from build123d import *

# Parameters (mm, degrees)
F0_R     = 1
F0_R_2   = 1.524
F1_DEPTH = 6.35


with BuildPart() as f1:
    # F0 (on Top) → F1 (new body)
    with BuildSketch(Plane.XY):
        with BuildLine():
            ThreePointArc((-196.395448, 36.447306), (-184.695448, -38.552694), (-196.395448, -113.552694))
            Line((-196.395448, -113.552694), (-146.395448, -113.552694))
            Line((-146.395448, -113.552694), (-146.395448, -73.552694))
            Line((-146.395448, -73.552694), (53.604552, -73.552694))
            Line((53.604552, -73.552694), (53.604552, -113.552694))
            Line((53.604552, -113.552694), (91.904552, -113.552694))
            ThreePointArc((91.904552, -113.552694), (103.604552, -38.552694), (91.904552, 36.447306))
            Line((91.904552, 36.447306), (65.304552, 36.447306))
            Line((65.304552, 36.447306), (53.604552, 36.447306))
            Line((53.604552, 36.447306), (53.604552, -3.552694))
            Line((53.604552, -3.552694), (-146.395448, -3.552694))
            Line((-146.395448, -3.552694), (-146.395448, 36.447306))
            Line((-146.395448, 36.447306), (-158.095448, 36.447306))
            Line((-158.095448, 36.447306), (-184.695448, 36.447306))
            Line((-184.695448, 36.447306), (-196.395448, 36.447306))
        make_face()
        with Locations((-180.445448, -109.302694)):
            Circle(F0_R, mode=Mode.SUBTRACT)
        with Locations((-162.345448, -109.302694)):
            Circle(F0_R, mode=Mode.SUBTRACT)
        with Locations((-164.375448, -62.682694)):
            Circle(F0_R_2, mode=Mode.SUBTRACT)
        with Locations((-112.305448, -57.602694)):
            Circle(F0_R_2, mode=Mode.SUBTRACT)
        with Locations((-81.825448, -62.682694)):
            Circle(F0_R_2, mode=Mode.SUBTRACT)
        with Locations((69.554552, -109.302694)):
            Circle(F0_R, mode=Mode.SUBTRACT)
        with Locations((87.654552, -109.302694)):
            Circle(F0_R, mode=Mode.SUBTRACT)
        with Locations((-163.105448, -14.422694)):
            Circle(F0_R_2, mode=Mode.SUBTRACT)
        with Locations((-112.305448, -29.662694)):
            Circle(F0_R_2, mode=Mode.SUBTRACT)
        with Locations((-88.175448, -14.422694)):
            Circle(F0_R_2, mode=Mode.SUBTRACT)
        with Locations((-180.445448, 32.197306)):
            Circle(F0_R, mode=Mode.SUBTRACT)
        with Locations((-162.345448, 32.197306)):
            Circle(F0_R, mode=Mode.SUBTRACT)
        with Locations((69.554552, 32.197306)):
            Circle(F0_R, mode=Mode.SUBTRACT)
        with Locations((87.654552, 32.197306)):
            Circle(F0_R, mode=Mode.SUBTRACT)
    extrude(amount=F1_DEPTH)


solid = f1.part
CAD build for the part. Positions are in the model's coordinates, mm. A direction names the side the tool comes from. Coordinates: 2 decimals unless noted, no trailing zeros. Loops run counter-clockwise (first coordinate to the right, second up) from the corner with the lowest first, then second, coordinate; pieces in that order, holes last. Notation, with made-up numbers: (28, 40) - (75, 40) arc R8 cw to (75, 51) - close; hole circle Ø11 at (86.5, -38.75). An arc over 180 degrees is marked (long way). Write item = value, one per line. Start each with the question number.
Q1. Drill centre lines: L1, parallel to Y at x = 32.5, z = 5.75; L2, parallel to X at y = -56.5, z = 2.25; L3, parallel to X at y = -93, z = 6.25. Where is each one in solid material? Low to high.
Q2. Pull direction X, two halves, no side cores. Call faces 4 (the flat face through (72, -113.553, 3)), 5 (the cylindrical face through (103.602, -39.62, 3.131)), 6 (the flat face through (-146.395, 16, 3)), 7 (the flat face through (-146.395, -94, 3)): pulls with the +X half, pulls with the -X half, needs draft (parallel to the pull), parting line crosses it, or undercut.
Q3. Cut at C-C, the plane x = -138.5. List the corners of the cut face in (y, z).
Q4. Cut at A-A, the plane z = 5. Give the number of separate pieces and of enclosed holes in the cut face, then the cut area to 3 significant figures.
Q5. Cut at D-D, the plane y = -49. List the corners of the cut face in (x, z).
Q6. Cut at B-B, the plane y = 22.5. List the corners of the cut face in (x, z).
Q7. Which spindle directions (+Z, -Z, +X, -X, +Y, -Y) get a long thin tool onto all of the face, cutting with end or side? Do faces 1 (the flat face through (-48, -38, 0)), 2 (the flat face through (-45, -3.553, 3)), 3 (the flat face through (53.605, -93, 3)). Say none if no direction does.
Q8. Flat gauge pins, fed straight in: pin 1 Ø1 at (y, z) = (-12, 5.5) entering from -X; pin 2 Ø3.5 at (x, y) = (-112.31, -29.66) entering from -Z; pin 3 Ø1 at (y, z) = (-81, 5) entering from -X; pin 4 Ø3 at (y, z) = (-70.5, 5.5) entering from +X. Where does each tip first touch, or does it go through?
Computed:
q1.L1 = -73.55 to -3.55
q1.L2 = -185.35 to -113.36, -111.25 to 102.95
q1.L3 = -190.79 to -146.4, 53.6 to 97.51
q2.face_4 = needs draft
q2.face_5 = pulls with the +X half
q2.face_6 = undercut
q2.face_7 = undercut
q3.outline = (-73.55, 0) - (-3.55, 0) - (-3.55, 6.35) - (-73.55, 6.35) - close
q4.separate_pieces = 1
q4.enclosed_holes = 14
q4.area = 27,200 mm²
q5.outline = (-184.92, 0) - (103.38, 0) - (103.38, 6.35) - (-184.92, 6.35) - close
q6.outline = (-192.38, 0) - (-146.4, 0) - (-146.4, 6.35) - (-192.38, 6.35) - close; (53.6, 0) - (95.92, 0) - (95.92, 6.35) - (53.6, 6.35) - close
q7.face_1 = -Z, +X, -X, +Y, -Y
q7.face_2 = +Z, -Z, +Y
q7.face_3 = +Z, -Z, -Y
q8.pin_1 = -186.19
q8.pin_2 = 0
q8.pin_3 = -188.47
q8.pin_4 = 101.71
